Input: part model. Units: mm. Frame: model coordinates. A direction names the side the tool comes from. Coordinates: 2 decimals unless noted, no trailing zeros. Order: outer loops, then holes, each group sorted by start corner. A loop starts at its lowest first (then second) coordinate and runs counter-clockwise, first axis right, second up. Notation, with made-up numbers: (18.5, 23) -> (58.5, 23) arc R17 cw to (58.5, 44) -> close; hole circle Ø9 at (27.5, 74). An arc over 180 degrees is marked (long way). Use one line per item in the form item = value. Start each with the question number.
1) Access query for faces 5 (the flat face through (-22.5, -2, -16)), 6 (the flat face through (0, 0, 5)), 7 (the flat face through (-21.514, 1.246, -15.776)), 8 (the flat face through (-12, 3, 1)), 9 (the flat face through (-20.5, 0, -16)). Directions: +Z, -Z, +X, -X, +Y, -Y. A direction counts if a zero-diameter tool reaches every point of the face in a straight line with its end or side. Return the directions, or none.
2) Section query D-D on z = 2. Output: boundary loops of the cut face in (x, y), then the cut area to 3 significant figures.
3) Section query B-B on x = -15.5. Output: boundary loops of the cut face in (y, z), then the cut area to 3 significant figures.
4) Section query C-C on y = 5.5. Output: boundary loops of the cut face in (x, z).
5) Section query A-A on z = -12. Output: boundary loops of the cut face in (x, y).
6) Ray query, line 1 along Y through (x, z) = (-15.5, 1); line 2 along Z through (x, y) = (14.5, -2.5); line 3 along X through (y, z) = (6.75, 11.5). Return the intervals inside material, ascending.
7) Draft query along X for faces 1 (the flat face through (-22.5, 2, -16)), 2 (the flat face through (27.5, 2, 14)), 3 (the cylindrical face through (-26.07, 0.04, 3.5)), 4 (the flat face through (25, 7, 11)). Return one class per face: pulls with the +X half, pulls with the -X half, needs draft (parallel to the pull), parting line crosses it, or undercut.
8) Pin query (flat end, axial travel): pin 1 (4 mm diameter, centred on x = 19, y = -1.5, fed in from +Z); pin 2 (2 mm diameter, centred on x = 12.5, y = 2, fed in from -Z); pin 3 (3 mm diameter, centred on y = 4, z = -9.5, fed in from -X); pin 4 (6 mm diameter, centred on y = 5.5, z = -17, fed in from +X). Return the tip coordinate at first contact, or that it passes through.
from build123d import *

# Parameters (mm, degrees)
SKETCH1_W           = 45
SKETCH1_H           = 6
BOSS_EXTRUDE1_DEPTH = 5
SKETCH2_W           = 37
SKETCH2_H           = 6
BOSS_EXTRUDE2_DEPTH = 5
FILLET1_R           = 5
SKETCH3_W           = 22
SKETCH3_H           = 10
BOSS_EXTRUDE3_DEPTH = 5
FILLET2_R           = 5
BOSS_EXTRUDE4_DEPTH = 32


with BuildPart() as part:
    # Sketch1 → Boss-Extrude1 (new body)
    with BuildSketch(Plane.XY):
        Rectangle(SKETCH1_W, SKETCH1_H)
    extrude(amount=BOSS_EXTRUDE1_DEPTH)

    # Sketch2 → Boss-Extrude2 (add)
    with BuildSketch(Plane.ZY.offset(22.5)):
        with Locations((-13.5, 0)):
            Rectangle(SKETCH2_W, SKETCH2_H)
    extrude(amount=BOSS_EXTRUDE2_DEPTH)

    # Fillet1
    fillet1_edges = [part.edges().sort_by_distance(p)[0] for p in [
        (-27.5, 0, 5),
    ]]
    fillet(fillet1_edges, radius=FILLET1_R)

    # Sketch3 → Boss-Extrude3 (add)
    with BuildSketch(Plane(origin=(22.5, 0, 0), x_dir=(0, 0, -1), z_dir=(1, 0, 0))):
        with Locations((-11, 2)):
            Rectangle(SKETCH3_W, SKETCH3_H)
    extrude(amount=BOSS_EXTRUDE3_DEPTH)

    # Fillet2
    fillet2_edges = [part.edges().sort_by_distance(p)[0] for p in [
        (27.5, 2, 0),
    ]]
    fillet(fillet2_edges, radius=FILLET2_R)

    # Sketch5 → Boss-Extrude4 (add)
    with BuildSketch(Plane(origin=(0, 0, 0), x_dir=(-1, 0, 0), z_dir=(0, 0, -1))):
        Polygon((22.5, 1), (20.5, 1.5), (20.5, -1.5), (22.5, -1), align=None)
    extrude(amount=BOSS_EXTRUDE4_DEPTH)


solid = part.part
Answers below:
q1.face_5 = -Z, -Y
q1.face_6 = +Z, -X, +Y, -Y
q1.face_7 = -Z, +Y
q1.face_8 = +Z, -Z, -X, +Y
q1.face_9 = -Z, +X, +Y, -Y
q2.outline = (-27.08, -3) -> (26.5, -3) -> (26.5, 7) -> (22.5, 7) -> (22.5, 3) -> (-27.08, 3) -> close
q2.area = 337 mm^2
q3.outline = (-3, 0) -> (3, 0) -> (3, 5) -> (-3, 5) -> close
q3.area = 30.0 mm^2
q4.outline = (22.5, 0) arc R5 ccw to (27.5, 5) -> (27.5, 22) -> (22.5, 22) -> close
q5.outline = (-27.5, -3) -> (-22.5, -3) -> (-22.5, -1) -> (-20.5, -1.5) -> (-20.5, 1.5) -> (-22.5, 1) -> (-22.5, 3) -> (-27.5, 3) -> close
q6.line_1 = -3 to 3
q6.line_2 = 0 to 5
q6.line_3 = 22.5 to 27.5
q7.face_1 = undercut
q7.face_2 = pulls with the +X half
q7.face_3 = pulls with the -X half
q7.face_4 = needs draft
q8.pin_1 = 5
q8.pin_2 = 0
q8.pin_3 = -27.5
q8.pin_4 = -22.5
